Verification items for the finished model (mm, model axes). Face numbers are marked on the shaded views. A direction names the side the tool comes from. Coordinates: 2 decimals unless noted, no trailing zeros. Write each loop counter-clockwise with the first axis right and the second up, starting at its lowest first coordinate (ties: lowest second). Pieces come first, ordered by that corner, then holes. Notation, with made-up numbers: (75.25, -11.75) -> (125.25, -11.75) arc R21 cw to (125.25, 8.25) -> close; hole circle Ø7 at (79.25, 72). An arc over 180 degrees is marked (long way). Answer in a Markdown table with one row per item.
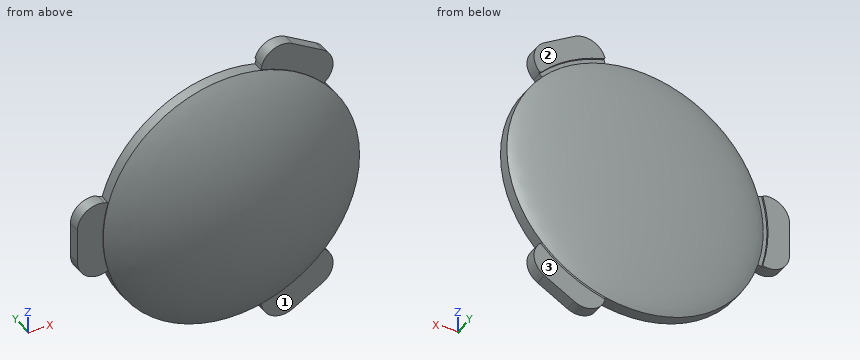
```python
from build123d import *

# Parameters (mm, degrees)
F0_W          = 17
F0_H          = 1.5
F3_DEPTH      = 0.75
F3_DEPTH_BACK = 0.65
F4_DEPTH      = 1
F5_T1_DEPTH   = 0.7858762015
F6_COUNT      = 3
F6_ANGLE      = 240


# Not quite as in the source:
# - a fillet or chamfer that OpenCascade refuses, or shapes differently, is made with other operations: its cross-section is extruded or revolved along the edge and cut away or added
# - a feature names something its author has since deleted; it is built from what else it names


with BuildPart() as f1:
    # F0 (on Top) → F1 (revolve)
    with BuildSketch(Plane.XY):
        with BuildLine():
            Line((0, 2.9235986368), (0, 0.75))
            Line((0, 0.75), (17, 0.75))
            add(Edge.make_bspline(
                [(17, 0.75), (14.7452850491, 2.0917814691), (7.445672527, 2.9235986368), (0, 2.9235986368)],
                knots=[0, 0, 0, 0, 17.1383934788, 17.1383934788, 17.1383934788, 17.1383934788], degree=3))
        make_face()
        with Locations((8.5, 0)):
            Rectangle(F0_W, F0_H)
        with BuildLine():
            Line((17, -0.75), (0, -0.75))
            Line((0, -0.75), (0, -5.8664013632))
            add(Edge.make_bspline(
                [(17, -0.75), (13.8637118638, -3.1852589455), (7.4548930861, -5.8664013632), (0, -5.8664013632)],
                knots=[0, 0, 0, 0, 17.7532409128, 17.7532409128, 17.7532409128, 17.7532409128], degree=3))
        make_face()
    revolve(axis=Axis((0, 1.8367993184, 0), (0, 1, 0)))

    # F2 (on Front) → F3 (join, two sides)
    with BuildSketch(Plane.XZ) as f3_sk:
        with BuildLine():
            ThreePointArc((-16.7830230255, -4.9578360326), (-17.5, 0), (-16.7830230255, 4.9578360326))
            ThreePointArc((-16.7830230255, 4.9578360326), (-19.2347780947, 4.5186022412), (-20.3506106924, 2.2917329463))
            Line((-20.3506106924, 2.2917329463), (-20.3506106924, 0))
            Line((-20.3506106924, 0), (-20.3506106924, -2.2917329463))
            ThreePointArc((-20.3506106924, -2.2917329463), (-19.2347780947, -4.5186022412), (-16.7830230255, -4.9578360326))
        make_face()
        with BuildLine():
            ThreePointArc((-16.3035080819, -4.8161835745), (-17, 0), (-16.3035080819, 4.8161835745))
            Line((-16.3035080819, 4.8161835745), (-16.7830230255, 4.9578360326))
            ThreePointArc((-16.7830230255, 4.9578360326), (-17.5, 0), (-16.7830230255, -4.9578360326))
            Line((-16.7830230255, -4.9578360326), (-16.3035080819, -4.8161835745))
        make_face()
    extrude(amount=-F3_DEPTH)
    extrude(f3_sk.sketch, amount=F3_DEPTH_BACK)

    # F2 (on Front) → F4 (join)
    with BuildSketch(Plane.XZ):
        with BuildLine():
            ThreePointArc((-16.7830230255, -4.9578360326), (-17.5, 0), (-16.7830230255, 4.9578360326))
            ThreePointArc((-16.7830230255, 4.9578360326), (-19.2347780947, 4.5186022412), (-20.3506106924, 2.2917329463))
            Line((-20.3506106924, 2.2917329463), (-20.3506106924, 0))
            Line((-20.3506106924, 0), (-20.3506106924, -2.2917329463))
            ThreePointArc((-20.3506106924, -2.2917329463), (-19.2347780947, -4.5186022412), (-16.7830230255, -4.9578360326))
        make_face()
    extrude(amount=-F4_DEPTH)

    # F5: fillet of radius 0.2 on 2 edges, made by hand

    # F5_s2 → F5_t1 (cut)
    with BuildSketch(Plane.XZ.offset(-1.5358762015)):
        with BuildLine():
            ThreePointArc((-16.9907798648, -5.0105923048), (-16.8612192668, -4.9182617144), (-16.84003675, -4.7605842351))
            ThreePointArc((-16.84003675, -4.7605842351), (-16.8118191828, -4.8592937518), (-16.7830230255, -4.9578360326))
            ThreePointArc((-16.7830230255, -4.9578360326), (-16.8863927879, -4.9862172864), (-16.9907798648, -5.0105923048))
        make_face()
        with BuildLine():
            ThreePointArc((-16.9907798648, 5.0105923048), (-16.8612192668, 4.9182617144), (-16.84003675, 4.7605842351))
            ThreePointArc((-16.84003675, 4.7605842351), (-16.8118191828, 4.8592937518), (-16.7830230255, 4.9578360326))
            ThreePointArc((-16.7830230255, 4.9578360326), (-16.8863927879, 4.9862172864), (-16.9907798648, 5.0105923048))
        make_face()
    extrude(amount=F5_T1_DEPTH, mode=Mode.SUBTRACT)

    # F6: F1 ×3 about axis
    f6_axis = Axis((0, -3.3082006816, 0), (0, -1, 0))


with BuildPart() as f1_1:
    add(f1.part)
    for i in range(1, F6_COUNT):
        add(f1.part.rotate(f6_axis, i * F6_ANGLE / (F6_COUNT - 1)))


solid = f1_1.part
```
1. Section check A-A, the plane y = 0.25. Record the boundary of the cut face in (x, z), plus the area to 3 significant figures.
Geometry says:
| item | result |
|---|---|
| outline | (-20.35, -2.29) arc R2.78 ccw to (-16.78, -4.96) -> (-16.3, -4.82) arc R17 ccw to (3.98, -16.53) -> (4.1, -17.01) arc R2.78 ccw to (8.19, -18.77) -> (12.16, -16.48) arc R2.78 ccw to (12.69, -12.06) -> (12.32, -11.71) arc R17 ccw to (12.32, 11.71) -> (12.69, 12.06) arc R2.78 ccw to (12.16, 16.48) -> (8.19, 18.77) arc R2.78 ccw to (4.1, 17.01) -> (3.98, 16.53) arc R17 ccw to (-16.3, 4.82) -> (-16.78, 4.96) arc R2.78 ccw to (-20.35, 2.29) -> close |
| area | 1,010 mm^2 |
2. Depth check by flat-ended pin: P1, Ø7.5, axis at x = 9.5, z = -15.5, coming from the +Y side; P2, Ø3, axis at x = -16.5, z = 8.5, coming from the +Y side; P3, Ø5, axis at x = -2.5, y = 1.5, coming from the -Z side; P4, Ø0.6, axis at x = -17, z = 0, coming from the +Y side. Enter the tip coordinate at first touch or a pass-through.
Geometry says:
| item | result |
|---|---|
| P1 | y = 1.66 |
| P2 | through |
| P3 | z = -17 |
| P4 | y = 0.91 |
3. Tool access check on the marked faces 1, 2 and 3. Record the directions out of +Z, -Z, +X, -X, +Y, -Y that give a thin tool (end or side, any length) a straight path to the whole face; none if there is none.
Geometry says:
| item | result |
|---|---|
| face 1 | -Z, +X, -Y |
| face 2 | +Z, +X, +Y |
| face 3 | -Z, +X, +Y |
4. Thickness scan on line 1 (Y direction, x = 5, z = 15); line 2 (Y direction, x = 14, z = 2.5); line 3 (Z direction, x = 7, y = 0.5). Record the ranges inside material, lowest first. Write a range as from..to.
Geometry says:
| item | result |
|---|---|
| line 1 | -1.58..1.27 |
| line 2 | -2.5..1.71 |
| line 3 | -19.14..19.14 |
